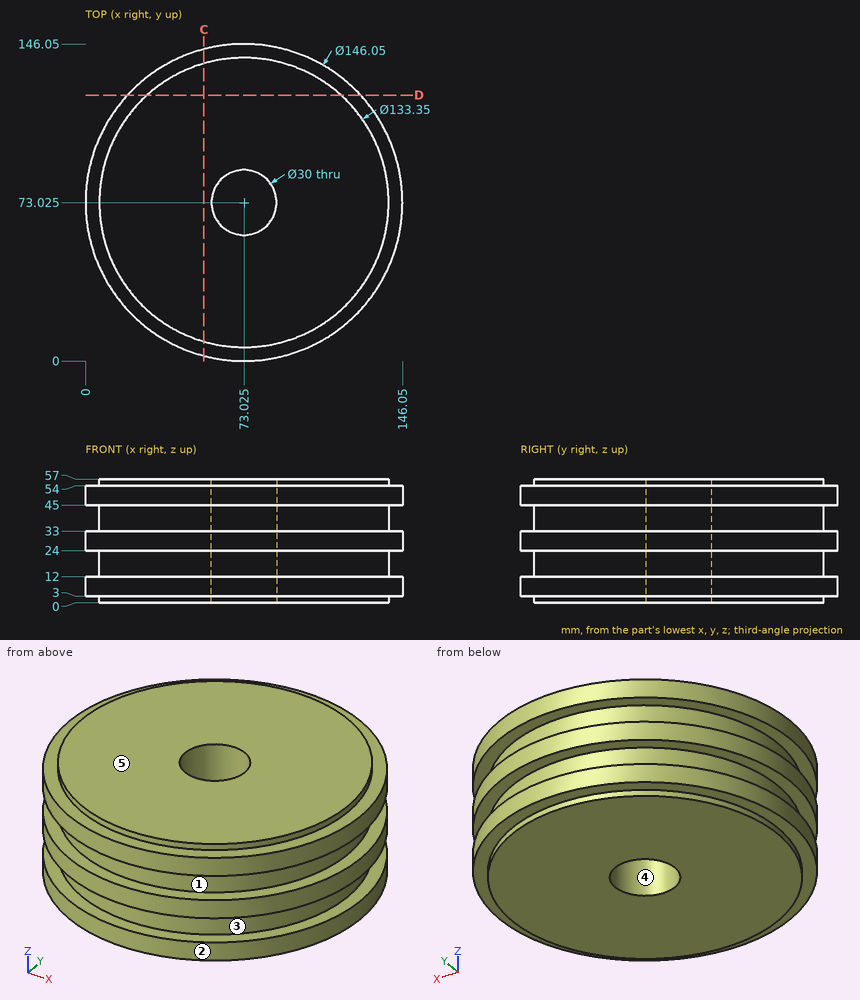
Study the drawing (mm; zero at the part's minimum x, y, z) and answer. A direction names the side the tool comes from. Coordinates: 2 decimals unless noted, no trailing zeros. Loops run counter-clockwise (first coordinate to the right, second up) from the corner with the lowest first, then second, coordinate; pieces in that order, holes last. Notation, with made-up numbers: (-37, 52.5) -> (-8, 52.5) arc R10 cw to (-8, 58.5) -> close; hole circle Ø6 at (21.5, 9.25). An arc over 180 degrees is marked (long way). Answer in a Markdown table with one row per item. Add a question column.
1. Consider line 1 (Z direction, x = 30, y = 15.5); line 2 (Y direction, x = 72.5, z = 52); line 3 (X direction, y = 62, z = 47.5). Determine where each line is inside the solid, lowest interval first. Write a range as [from, to].
2. The part is cut by section D-D, the plane y = 122.5. Write down the section's boundary in (x, z), then the cut area to 3 significant figures.
3. The part is cut by section C-C, the plane x = 54.5. Write down the section's boundary in (y, z), then the cut area to 3 significant figures.
4. Determine the mould class of the marked faces 3, 4 and 5 for opening direction Z: +Z half, -Z half, draft (parallel to the pull), parting line (faces both ways), or undercut.
5. Flat-ended cylindrical pins translate along their axes: P1, Ø1, axis at y = 81, z = 37, coming from the +X side; P2, Ø6, axis at x = 82, z = 31, coming from the +Y side; P3, Ø1, axis at x = 104, z = 11.5, coming from the -Y side. Find the tip coordinate at first contact, or state that the pin passes through.
6. For the marked faces 1 and 2, determine the directions among +Z, -Z, +X, -X, +Y, -Y from which every point of the face is accessible in a straight line to the end or side of a thin tool.
Answer below:
| question | item | result |
|---|---|---|
| 1 | line 1 | [3, 12], [24, 33], [45, 54] |
| 1 | line 2 | [0, 58.03], [88.02, 146.05] |
| 1 | line 3 | [0.84, 62.85], [83.2, 145.21] |
| 2 | outline | (19.31, 3) -> (28.33, 3) -> (28.33, 0) -> (117.72, 0) -> (117.72, 3) -> (126.74, 3) -> (126.74, 12) -> (117.72, 12) -> (117.72, 24) -> (126.74, 24) -> (126.74, 33) -> (117.72, 33) -> (117.72, 45) -> (126.74, 45) -> (126.74, 54) -> (117.72, 54) -> (117.72, 57) -> (28.33, 57) -> (28.33, 54) -> (19.31, 54) -> (19.31, 45) -> (28.33, 45) -> (28.33, 33) -> (19.31, 33) -> (19.31, 24) -> (28.33, 24) -> (28.33, 12) -> (19.31, 12) -> close |
| 2 | area | 5,580 mm2 |
| 3 | outline | (2.39, 3) -> (8.98, 3) -> (8.98, 0) -> (137.07, 0) -> (137.07, 3) -> (143.66, 3) -> (143.66, 12) -> (137.07, 12) -> (137.07, 24) -> (143.66, 24) -> (143.66, 33) -> (137.07, 33) -> (137.07, 45) -> (143.66, 45) -> (143.66, 54) -> (137.07, 54) -> (137.07, 57) -> (8.98, 57) -> (8.98, 54) -> (2.39, 54) -> (2.39, 45) -> (8.98, 45) -> (8.98, 33) -> (2.39, 33) -> (2.39, 24) -> (8.98, 24) -> (8.98, 12) -> (2.39, 12) -> close |
| 3 | area | 7,660 mm2 |
| 4 | face 3 | undercut |
| 4 | face 4 | draft |
| 4 | face 5 | +Z half |
| 5 | P1 | x = 139.28 |
| 5 | P2 | y = 145.81 |
| 5 | P3 | y = 6.66 |
| 6 | face 1 | none |
| 6 | face 2 | +Z, -Z |
